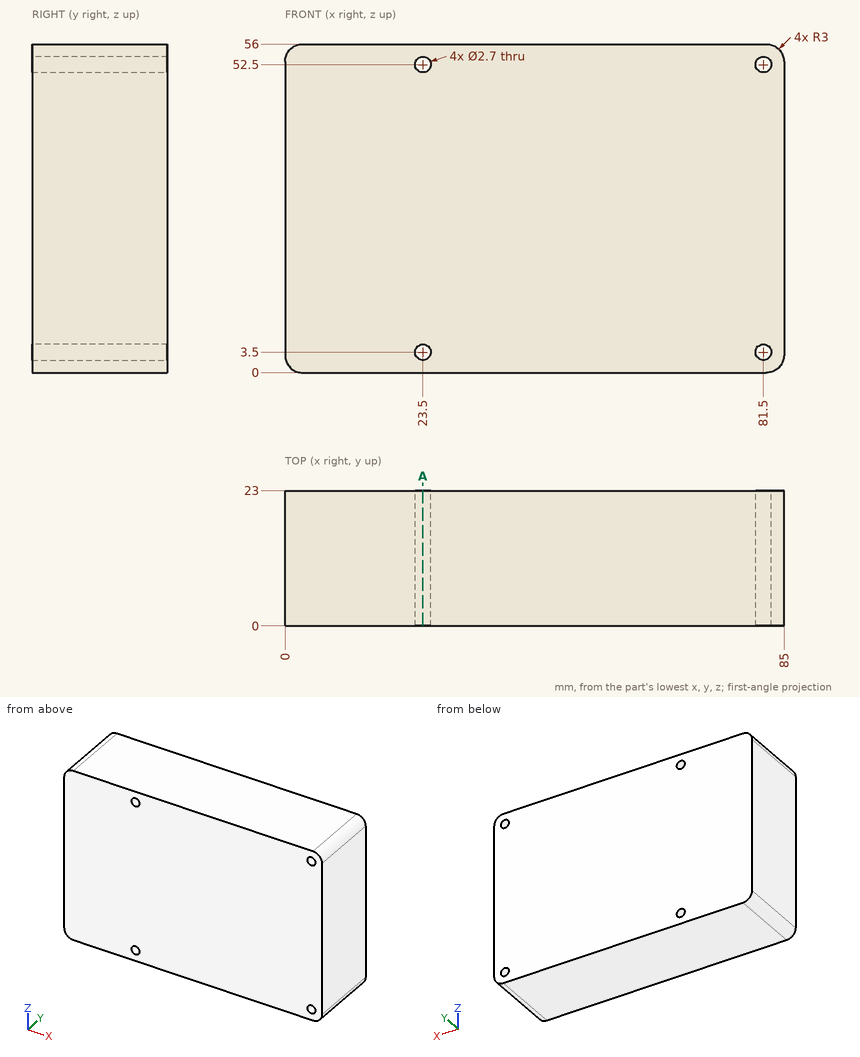
The figure shows three views and two pictorial views of one solid part (mm, origin at its lowest corner). Answer the questions. Coordinates: 2 decimals unless noted, no trailing zeros. Write each loop counter-clockwise with the first axis right and the second up, starting at its lowest first coordinate (ties: lowest second). Pieces come first, ordered by that corner, then holes.
1. Consider line 1 along X through (y, z) = (9.25, 52.5); line 2 along Z through (x, y) = (81.5, 16). Determine where each line is inside the solid, lowest interval first.
Results list:
line 1: x = 0 to 22.15, 24.85 to 80.15, 82.85 to 85
line 2: z = 0 to 2.15, 4.85 to 51.15, 53.85 to 56
2. The part is cut by section A-A, the plane x = 23.5. Write down the section's boundary in (y, z), and give its area (3 significant figures).
Results list:
outline: (0, 0) - (23, 0) - (23, 2.15) - (0, 2.15) - close; (0, 4.85) - (23, 4.85) - (23, 51.15) - (0, 51.15) - close; (0, 53.85) - (23, 53.85) - (23, 56) - (0, 56) - close
area: 1,160 mm2
3. A flat-ended cylindrical pin translates along its axis: pin 1 (1.5 mm diameter, centred on y = 11, z = 39, fed in from -X). Find the tip coordinate at first contact, or state that the pin passes through.
Results list:
pin 1: stops at x = 0
